Check sheet for the modelled part. Datum: model origin and axes. Units: mm. Face numbers are marked on the shaded views. Coordinates: 2 decimals unless noted, no trailing zeros. Write each loop counter-clockwise with the first axis right and the second up, starting at its lowest first coordinate (ties: lowest second). Pieces come first, ordered by that corner, then holes. Notation, with made-up numbers: M 8,2.25 L 55,2.25 A15 ccw 55,31.25 Z; hole C -10,74.5 d9. An arc over 180 degrees is marked long. Answer as CSV lines item,"result". Start each with the question number.
Q1. Sectioned sample at D-D, the plane x = 62. Record the cut outline in (y, z), then the cut area to 3 significant figures.
Q2. Thickness scan on line 1 along Y through (x, z) = (31, -32); line 2 along Z through (x, y) = (-68, -78.5); line 3 along X through (y, z) = (3, 39). Record the ranges inside material, lowest first. Write a range as from..to.
Q3. Sectioned sample at C-C, the plane z = 39.5. Record the cut outline in (x, y), then the cut area to 3 significant figures.
Q4. Sectioned sample at A-A, the plane x = -1. Record the cut outline in (y, z), then the cut area to 3 significant figures.
Q5. Depth check by flat-ended pin: pin 1 Ø12 at (x, y) = (-58, -84.5) entering from +Z; pin 2 Ø4 at (y, z) = (-4.5, -55.5) entering from +X; pin 3 Ø1.5 at (x, z) = (55, -22) entering from -Y. Enter the tip coordinate at first touch or a pass-through.
Q6. Mould release check, pull along Z, two halves, no side actions. Record for the marked faces 1 and 2: pulls with the +Z half, pulls with the -Z half, needs draft (parallel to the pull), parting line crosses it, or undercut.
Q7. Sectioned sample at B-B, the plane y = -78.5. Record the cut outline in (x, z).
from build123d import *

# Parameters (mm, degrees)
SKETCH1_W           = 150
SKETCH1_H           = 150
BOSS_EXTRUDE2_DEPTH = 10
BOSS_EXTRUDE3_DEPTH = 100
SKETCH4_W           = 42
SKETCH4_H           = 65
CUT_EXTRUDE1_DEPTH  = 111


with BuildPart() as part:
    # Sketch1 → Boss-Extrude2 (new body)
    with BuildSketch(Plane(origin=(0, 0, 0), x_dir=(1, 0, 0), z_dir=(0, 1, 0))):
        Rectangle(SKETCH1_W, SKETCH1_H)
    extrude(amount=BOSS_EXTRUDE2_DEPTH)

    # Sketch3 → Boss-Extrude3 (add)
    with BuildSketch(Plane.XZ):
        with BuildLine():
            ThreePointArc((-59, 65), (-69.242640687, 69.242640687), (-65, 59))
            Line((-65, 59), (-65, 65))
            Line((-65, 65), (-59, 65))
        make_face()
        with BuildLine():
            Line((-65, 65), (-65, 59))
            ThreePointArc((-65, 59), (-60.757359313, 60.757359313), (-59, 65))
            Line((-59, 65), (-65, 65))
        make_face()
        with BuildLine():
            ThreePointArc((59, 65), (60.757359313, 60.757359313), (65, 59))
            Line((65, 59), (65, 65))
            Line((65, 65), (59, 65))
        make_face()
        with BuildLine():
            Line((65, 65), (65, 59))
            ThreePointArc((65, 59), (69.242640687, 60.757359313), (71, 65))
            ThreePointArc((71, 65), (65, 71), (59, 65))
            Line((59, 65), (65, 65))
        make_face()
        with BuildLine():
            ThreePointArc((59, 65), (60.757359313, 60.757359313), (65, 59))
            Line((65, 59), (65, 65))
            Line((65, 65), (59, 65))
        make_face()
        with BuildLine():
            Line((65, 65), (65, 59))
            ThreePointArc((65, 59), (69.242640687, 60.757359313), (71, 65))
            ThreePointArc((71, 65), (65, 71), (59, 65))
            Line((59, 65), (65, 65))
        make_face()
        with BuildLine():
            ThreePointArc((-59, 65), (-69.242640687, 69.242640687), (-65, 59))
            Line((-65, 59), (-65, 65))
            Line((-65, 65), (-59, 65))
        make_face()
        with BuildLine():
            Line((-65, 65), (-65, 59))
            ThreePointArc((-65, 59), (-60.757359313, 60.757359313), (-59, 65))
            Line((-59, 65), (-65, 65))
        make_face()
        with BuildLine():
            Line((-65, -59), (-65, -65))
            Line((-65, -65), (-59, -65))
            ThreePointArc((-59, -65), (-60.757359313, -60.757359313), (-65, -59))
        make_face()
        with BuildLine():
            Line((-59, -65), (-65, -65))
            Line((-65, -65), (-65, -59))
            ThreePointArc((-65, -59), (-69.242640687, -69.242640687), (-59, -65))
        make_face()
        with BuildLine():
            Line((-65, -59), (-65, -65))
            Line((-65, -65), (-59, -65))
            ThreePointArc((-59, -65), (-60.757359313, -60.757359313), (-65, -59))
        make_face()
        with BuildLine():
            Line((-59, -65), (-65, -65))
            Line((-65, -65), (-65, -59))
            ThreePointArc((-65, -59), (-69.242640687, -69.242640687), (-59, -65))
        make_face()
        with BuildLine():
            ThreePointArc((65, -59), (60.757359313, -60.757359313), (59, -65))
            Line((59, -65), (65, -65))
            Line((65, -65), (65, -59))
        make_face()
        with BuildLine():
            Line((65, -65), (59, -65))
            ThreePointArc((59, -65), (65, -71), (71, -65))
            ThreePointArc((71, -65), (69.242640687, -60.757359313), (65, -59))
            Line((65, -59), (65, -65))
        make_face()
        with BuildLine():
            ThreePointArc((65, -59), (60.757359313, -60.757359313), (59, -65))
            Line((59, -65), (65, -65))
            Line((65, -65), (65, -59))
        make_face()
        with BuildLine():
            Line((65, -65), (59, -65))
            ThreePointArc((59, -65), (65, -71), (71, -65))
            ThreePointArc((71, -65), (69.242640687, -60.757359313), (65, -59))
            Line((65, -59), (65, -65))
        make_face()
    extrude(amount=BOSS_EXTRUDE3_DEPTH)

    # Sketch4 → Cut-Extrude1 (cut, through all)
    with BuildSketch(Plane(origin=(0, 10, 0), x_dir=(1, 0, 0), z_dir=(0, 1, 0))):
        with Locations((0, -17.25)):
            Rectangle(SKETCH4_W, SKETCH4_H)
    extrude(amount=-CUT_EXTRUDE1_DEPTH, mode=Mode.SUBTRACT)


solid = part.part
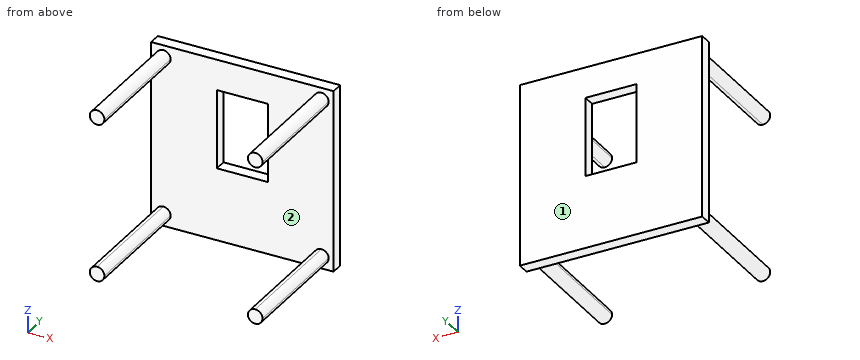
Output:
1,outline,"M -100,-70.2 L 0,-70.2 L 0,-75 L 10,-75 L 10,75 L 0,75 L 0,70.2 L -100,70.2 L -100,59.8 L 0,59.8 L 0,-59.8 L -100,-59.8 Z"
1,area,"3,580 mm^2"
2,line 1,"y = 0..10"
2,line 2,"z = -70.2..-59.8, 59.8..70.2"
2,line 3,"x = -75..-21, 21..75"
3,outline,"M -75,0 L -21,0 L -21,10 L -75,10 Z; M 21,0 L 75,0 L 75,10 L 21,10 Z"
3,area,"1,080 mm^2"
4,outline,"M 0,-75 L 10,-75 L 10,-15.25 L 0,-15.25 Z; M 0,49.75 L 10,49.75 L 10,75 L 0,75 Z"
4,area,"850 mm^2"
5,pin 1,"stops at z = 70.92"
5,pin 2,"passes through"
5,pin 3,"stops at y = 0"
6,face 1,"needs draft"
6,face 2,"undercut"
7,outline,"C -65,-65 d12; C -65,65 d12; C 65,-65 d12; C 65,65 d12"
